```python
from build123d import *

# Parameters (mm, degrees)
SKETCH1_R           = 15
BOSS_EXTRUDE1_DEPTH = 10
SKETCH2_R           = 8
CUT_EXTRUDE1_DEPTH  = 5
CUT_EXTRUDE2_REACH  = 25.452


with BuildPart() as part:
    # Sketch1 → Boss-Extrude1 (new body)
    with BuildSketch(Plane(origin=(0, 0, 0), x_dir=(1, 0, 0), z_dir=(0, 1, 0))):
        with Locations(Location((0, 0, 0), (0, 0, 270))):
            Circle(SKETCH1_R)
    extrude(amount=BOSS_EXTRUDE1_DEPTH)

    # Sketch2 → Cut-Extrude1 (cut)
    with BuildSketch(Plane(origin=(0, 10, 0), x_dir=(1, 0, 0), z_dir=(0, 1, 0))):
        with Locations(Location((0, 0, 0), (0, 0, 270))):
            Circle(SKETCH2_R)
    extrude(amount=-CUT_EXTRUDE1_DEPTH, mode=Mode.SUBTRACT)

    # Sketch3 → Cut-Extrude2 (cut, up to next)
    with BuildSketch(Plane(origin=(0, 10, 0), x_dir=(1, 0, 0), z_dir=(0, 1, 0)), mode=Mode.PRIVATE) as cut_extrude2_sk1:
        Polygon((-4.993128311, 14.139704236), (-4.993128311, 16.53849836), (5.006871689, 16.53849836), (5.006871689, 14.139704236), (5.006871689, 11.139704236), (-4.993128311, 11.139704236), align=None)
    cut_extrude2_tool1 = extrude(cut_extrude2_sk1.sketch, amount=-CUT_EXTRUDE2_REACH, mode=Mode.PRIVATE) & part.part
    # Sketch3 → Cut-Extrude2 (cut, up to next)
    with BuildSketch(Plane(origin=(0, 10, 0), x_dir=(1, 0, 0), z_dir=(0, 1, 0)), mode=Mode.PRIVATE) as cut_extrude2_sk2:
        Polygon((9.741907226, -11.405930195), (7.143831014, -9.905930195), (12.143831014, -1.245676157), (14.741907226, -2.745676157), (16.819323876, -3.945073219), (11.819323876, -12.605327257), align=None)
    cut_extrude2_tool2 = extrude(cut_extrude2_sk2.sketch, amount=-CUT_EXTRUDE2_REACH, mode=Mode.PRIVATE) & part.part
    # Sketch3 → Cut-Extrude2 (cut, up to next)
    with BuildSketch(Plane(origin=(0, 10, 0), x_dir=(1, 0, 0), z_dir=(0, 1, 0)), mode=Mode.PRIVATE) as cut_extrude2_sk3:
        Polygon((-14.748778915, -2.733774042), (-12.150702704, -1.233774042), (-7.150702704, -9.894028079), (-9.748778915, -11.394028079), (-11.826195565, -12.593425141), (-16.826195565, -3.933171104), align=None)
    cut_extrude2_tool3 = extrude(cut_extrude2_sk3.sketch, amount=-CUT_EXTRUDE2_REACH, mode=Mode.PRIVATE) & part.part
    add(cut_extrude2_tool1.solids().sort_by_distance((0.006872, 10, -13.839101))[0], mode=Mode.SUBTRACT)
    add(cut_extrude2_tool2.solids().sort_by_distance((11.981577, 10, 6.925502))[0], mode=Mode.SUBTRACT)
    add(cut_extrude2_tool3.solids().sort_by_distance((-11.988449, 10, 6.9136))[0], mode=Mode.SUBTRACT)


solid = part.part
```
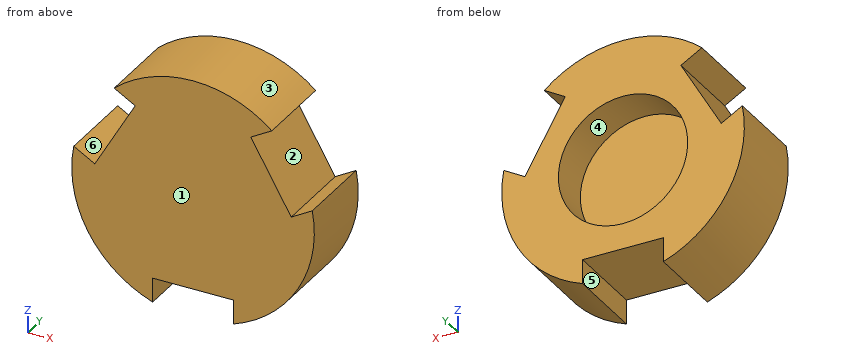
Here's how the part is built. I have some questions about the finished solid (model axes, mm). Face numbers are marked on the shaded views. A direction names the side the tool comes from. Give positions to 0.01 mm unless a question says otherwise; leave off trailing zeros. Write each loop counter-clockwise with the first axis right and the second up, starting at its lowest first coordinate (ties: lowest second). Pieces come first, ordered by that corner, then holes. Notation, with made-up numbers: M 64.5,83.25 L 119.5,83.25 A20 cw 119.5,105.25 Z; hole C 26.5,10 d9. An arc over 180 degrees is marked long. Put each result on its own line as item: value. Start each with the question number.
Item 1: Will these pins go through, and if not, where does the flat tip stop? pin 1 (0.9 mm diameter, centred on y = 5, z = -12.5, fed in from -X); pin 2 (1.5 mm diameter, centred on y = 2.5, z = -5.5, fed in from -X); pin 3 (4 mm diameter, centred on y = 7, z = -1.5, fed in from -X); pin 4 (1 mm diameter, centred on y = 8.5, z = -1.5, fed in from +X).
Item 2: If we section it at B-B, the plane z = 0: Write out the boundary of the cut face in (x, y).
Item 3: On a 3-axis mill with a long thin cutter (end or side, diameter ignored), from which of +Z, -Z, +X, -X, +Y, -Y can I reach the whole of each face in a straight line? I mean the marked faces 4, 5 and 6. Say none if no direction works.
Item 4: If we section it at A-A, the plane y = 8: Write out the boundary of the cut face in (x, z).
Item 5: Thinking about a two-plate mould opening in Z: for the marked faces 1, 2 and 3, which applies, +Z half, -Z half, draft (parallel to the pull), parting line (faces both ways), or undercut?
Item 6: If we section it at C-C, the plane y = 2: Write out the boundary of the cut face in (x, z).
Item 7: If we section it at D-D, the plane x = -9: Write out the boundary of the cut face in (y, z), then the cut area to 3 significant figures.
Item 8: I need wall thicknesses on L1, parallel to X at y = 7.1, z = 0; L2, parallel to X at y = 7.5, z = 2.5; L3, parallel to Y at x = -1, z = -6.5. Which ranges of each line are inside material? Lowest first, please. Write a range as from..to.
Values:
1. pin 1: x = -8.93
1. pin 2: x = -14.23
1. pin 3: x = -15
1. pin 4: x = 14.97
2. outline: M -15,0 L 15,0 L 15,10 L 8,10 L 8,5 L -8,5 L -8,10 L -15,10 Z
3. face 4: +Y
3. face 5: -Z, +Y, -Y
3. face 6: +Z, +Y, -Y
4. outline: M -14.75,2.73 A15 ccw -4.99,-14.14 L -4.99,-11.14 L 5.01,-11.14 L 5.01,-14.14 A15 ccw 14.75,2.75 L 12.14,1.25 L 7.14,9.91 L 9.74,11.41 A15 ccw -9.75,11.4 L -7.15,9.89 L -12.15,1.23 Z; hole C 0,0 d16
5. face 1: draft
5. face 2: undercut
5. face 3: +Z half
6. outline: M -14.75,2.73 A15 ccw -4.99,-14.14 L -4.99,-11.14 L 5.01,-11.14 L 5.01,-14.14 A15 ccw 14.75,2.75 L 12.14,1.25 L 7.14,9.91 L 9.74,11.41 A15 ccw -9.75,11.4 L -7.15,9.89 L -12.15,1.23 Z
7. outline: M 0,-12 L 10,-12 L 10,6.69 L 0,6.69 Z; M 0,10.96 L 10,10.96 L 10,12 L 0,12 Z
7. area: 197 mm²
8. L1: -15..-8, 8..15
8. L2: -14.79..-14.34, -11.42..-7.6, 7.6..11.42, 14.32..14.79
8. L3: 0..5
